from build123d import *

# Parameters (mm, degrees)
BOSS_EXTRUDE2_DEPTH = 3.175
SKETCH3_R           = 1.7
CUT_EXTRUDE2_DEPTH  = 3.175
SKETCH4_R           = 1.5
CUT_EXTRUDE3_DEPTH  = 3.175
SKETCH5_W           = 61.765088801
SKETCH5_H           = 64
CUT_EXTRUDE4_DEPTH  = 3.175
FILLET1_R           = 2


with BuildPart() as part:
    # Sketch1 → Boss-Extrude2 (new body)
    with BuildSketch(Plane(origin=(0, 0, 0), x_dir=(1, 0, 0), z_dir=(0, 1, 0))):
        with BuildLine():
            Line((-22, 32), (22, 32))
            ThreePointArc((22, 32), (29.071067812, 29.071067812), (32, 22))
            Line((32, 22), (32, -22))
            ThreePointArc((32, -22), (29.071067812, -29.071067812), (22, -32))
            Line((22, -32), (-22, -32))
            ThreePointArc((-22, -32), (-29.071067812, -29.071067812), (-32, -22))
            Line((-32, -22), (-32, 22))
            ThreePointArc((-32, 22), (-29.071067812, 29.071067812), (-22, 32))
        make_face()
    extrude(amount=BOSS_EXTRUDE2_DEPTH)

    # Sketch3 → Cut-Extrude2 (cut)
    with BuildSketch(Plane(origin=(0, 3.175, 0), x_dir=(1, 0, 0), z_dir=(0, 1, 0))):
        with Locations((-23.5, 23.5)):
            Circle(SKETCH3_R)
        with Locations((23.5, 23.5)):
            Circle(SKETCH3_R)
        with Locations((23.5, -23.5)):
            Circle(SKETCH3_R)
        with Locations((-23.5, -23.5)):
            Circle(SKETCH3_R)
    extrude(amount=-CUT_EXTRUDE2_DEPTH, mode=Mode.SUBTRACT)

    # Sketch4 → Cut-Extrude3 (cut)
    with BuildSketch(Plane(origin=(0, 3.175, 0), x_dir=(1, 0, 0), z_dir=(0, 1, 0))):
        with Locations((24, -5)):
            Circle(SKETCH4_R)
        with Locations((-24, -5)):
            Circle(SKETCH4_R)
    extrude(amount=-CUT_EXTRUDE3_DEPTH, mode=Mode.SUBTRACT)

    # Sketch5 → Cut-Extrude4 (cut)
    with BuildSketch(Plane(origin=(0, 3.175, 0), x_dir=(1, 0, 0), z_dir=(0, 1, 0))):
        with Locations((-13.882544401, 0)):
            Rectangle(SKETCH5_W, SKETCH5_H)
    extrude(amount=-CUT_EXTRUDE4_DEPTH, mode=Mode.SUBTRACT)

    # Fillet1
    fillet1_edges = [part.edges().sort_by_distance(p)[0] for p in [
        (17, 1.5875, 32),
        (17, 1.5875, -32),
    ]]
    fillet(fillet1_edges, radius=FILLET1_R)


solid = part.part
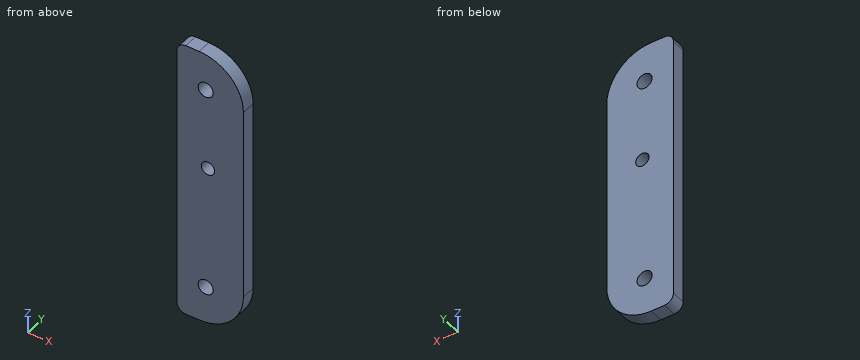
Design review of the part built by this model. Coordinates are the model's own, in mm. Round coordinates to 2 decimals unless told otherwise and drop trailing zeros. Write each loop counter-clockwise with the first axis right and the second up, starting at its lowest first coordinate (ties: lowest second). Pieces come first, ordered by that corner, then holes. Notation, with made-up numbers: (33.5, -20) -> (52.5, -20) arc R10 cw to (52.5, -2) -> close; hole circle Ø10 at (-8, -2). An arc over 180 degrees is marked (long way). One line per question, with ' | ' between items.
(1) Take a section at C-C, the plane x = 24.5. State the section outline as (y, z) points (3 decimals).
Result sheet:
outline: (0, -31.682) -> (3.175, -31.682) -> (3.175, -24.875) -> (0, -24.875) -> close; (0, -22.125) -> (3.175, -22.125) -> (3.175, 3.586) -> (0, 3.586) -> close; (0, 6.414) -> (3.175, 6.414) -> (3.175, 22.125) -> (0, 22.125) -> close; (0, 24.875) -> (3.175, 24.875) -> (3.175, 31.682) -> (0, 31.682) -> close
(2) Take a section at D-D, the plane z = -23.5. State the section outline as (x, y) points (3 decimals), and give its area (3 significant figures).
Result sheet:
outline: (17, 0) -> (21.8, 0) -> (21.8, 3.175) -> (17, 3.175) -> close; (25.2, 0) -> (31.887, 0) -> (31.887, 3.175) -> (25.2, 3.175) -> close | area: 36.5 mm2
(3) Wall thickness on line 1 (Z direction, x = 25, y = 2.9); line 2 (Z direction, x = 24, y = 0.7); line 3 (Z direction, x = 28, y = 0.25): over which ranges is each line inside the solid? List them lowest first. Write a range as [from, to].
Result sheet:
line 1: [-31.54, -24.3], [-22.7, 3.88], [6.12, 22.7], [24.3, 31.54] | line 2: [-31.8, -25.12], [-21.88, 3.5], [6.5, 21.88], [25.12, 31.8] | line 3: [-30, 30]
(4) Take a section at B-B, the plane y = 1.3. State the section outline as (x, z) points.
Result sheet:
outline: (17, -30) arc R2 ccw to (19, -32) -> (22, -32) arc R10 ccw to (32, -22) -> (32, 22) arc R10 ccw to (22, 32) -> (19, 32) arc R2 ccw to (17, 30) -> close; hole circle Ø3.4 at (23.5, -23.5); hole circle Ø3.4 at (23.5, 23.5); hole circle Ø3 at (24, 5)
(5) Take a section at A-A, the plane z = 5. State the section outline as (x, y) points (3 decimals).
Result sheet:
outline: (17, 0) -> (22.5, 0) -> (22.5, 3.175) -> (17, 3.175) -> close; (25.5, 0) -> (32, 0) -> (32, 3.175) -> (25.5, 3.175) -> close
